For this review, take the finished solid that the model builds, in its own axes (mm). A direction names the side the tool comes from. Give positions to 0.01 mm unless a question says otherwise; leave off trailing zeros. Order: outer loops, then holes, each group sorted by start corner. A loop starts at its lowest first (then second) coordinate and runs counter-clockwise, first axis right, second up.
from build123d import *

# Parameters (mm, degrees)
SKETCH1_W          = 33.5
SKETCH1_H          = 1.1
CUT_EXTRUDE1_DEPTH = 1
SCALE1_SCALE       = 2


with BuildPart() as part:
    # Sketch1 → Revolve1 (revolve)
    with BuildSketch(Plane.XY):
        with Locations((4.269842451, 0.55)):
            Rectangle(SKETCH1_W, SKETCH1_H)
        with BuildLine():
            Line((-12.830157549, 0), (-12.830157549, 2.85))
            ThreePointArc((-12.830157549, 2.85), (-13.77738043, 2.26408121), (-14.480157549, 1.4))
            Line((-14.480157549, 1.4), (-14.480157549, 0))
            Line((-14.480157549, 0), (-12.830157549, 0))
        make_face()
        Polygon((-12.480157549, 1.1), (-12.480157549, 2.85), (-12.830157549, 2.85), (-12.830157549, 0), (-12.480157549, 0), align=None)
        Polygon((21.319842451, 0.8), (21.019842451, 1.1), (21.019842451, 0), (21.319842451, 0), align=None)
    revolve(axis=Axis((-12.480157549, 0, 0), (1, 0, 0)))

    # Sketch2 → Cut-Extrude1 (cut)
    with BuildSketch(Plane.ZY.offset(14.480157549)):
        Polygon((0, 1.154700538), (-1, 0.577350269), (-1, -0.577350269), (0, -1.154700538), (1, -0.577350269), (1, 0.577350269), align=None)
    extrude(amount=-CUT_EXTRUDE1_DEPTH, mode=Mode.SUBTRACT)


with BuildPart() as part_1:
    # Scale1: scaled about (0.733669991, 0, 0)
    add(part.part.scale(SCALE1_SCALE).moved(Location((-0.733669991, 0, 0))))


solid = part_1.part
1) Tool access review of faces 1 (the face through (41.906, 0, 0)), 2 (the face through (-25.694, 0.1, -2.5)), 3 (the face through (-29, 0, 2)): name each direction out of +Z, -Z, +X, -X, +Y, -Y from which nothing blocks a thin tool from reaching the whole face with its end or side.
Answer sheet:
face 1: +Z, -Z, +X, +Y, -Y
face 2: +X
face 3: -X
2) Clearance check with flat-ended pins moving along their axes: pin 1 (3 mm diameter, centred on y = 3, z = -4.5, fed in from -X); pin 2 (1 mm diameter, centred on x = -28.5, y = 0.5, fed in from -Z); pin 3 (1 mm diameter, centred on x = 29.5, z = 1, fed in from +Y). State where each tip first meets the part, or that it passes through.
Answer sheet:
pin 1: stops at x = -28.91
pin 2: stops at z = -4.74
pin 3: stops at y = 2.14
3) To check wall thickness, follow line 1 (Y direction, x = -21, z = 0.25); line 2 (X direction, y = -0.5, z = -0.25); line 3 (Z direction, x = -21, y = 1.5). State the ranges of each line that lie inside material, in increasing order.
Answer sheet:
line 1: y = -2.19 to 2.19
line 2: x = -27.69 to 41.91
line 3: z = -1.61 to 1.61
4) Draft analysis for pull direction Y (two halves, no side actions). For faces 4 (the face through (-26, -4.5, -3.5)), 5 (the face through (-28.71, -1.74, 0.99)), 6 (the face through (-27.694, 0, 0)), 7 (the face through (-29.694, -2, -1)), state which applies: +Y half, -Y half, draft (parallel to the pull), parting line (faces both ways), or undercut.
Answer sheet:
face 4: parting line
face 5: undercut
face 6: undercut
face 7: draft
5) We need section A-A on x = 9. Give the boundary of the cut face in (y, z).
Answer sheet:
outline: circle Ø4.4 at (0, 0)
